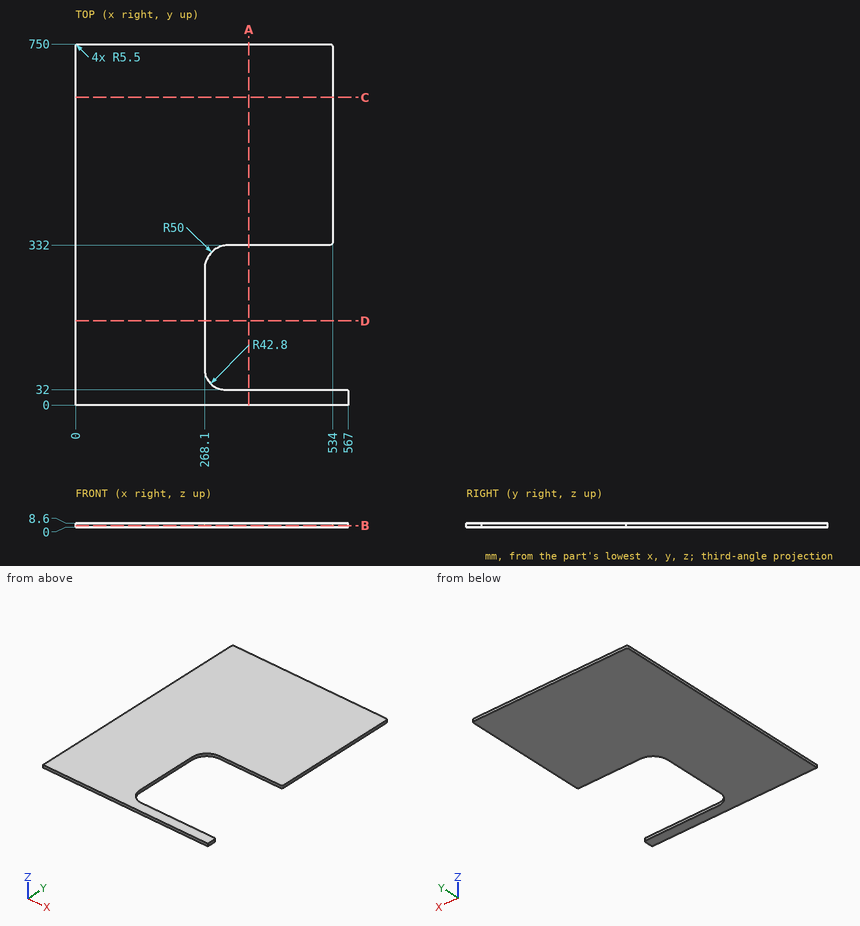
Print and shaded views of the part. All mm, measured from the part's lowest x, y and z. Coordinates: 2 decimals unless noted, no trailing zeros. Order: outer loops, then holes, each group sorted by start corner. A loop starts at its lowest first (then second) coordinate and runs counter-clockwise, first axis right, second up.
Item 1: Drill centre lines: L1, parallel to Y at x = 348, z = 6.75; L2, parallel to X at y = 92, z = 6.5; L3, parallel to X at y = 350, z = 7.5. Where is each one in solid material? Low to high.
Filled in:
L1: y = 0 to 32, 332 to 750
L2: x = 0 to 268.1
L3: x = 0 to 534
Item 2: Saw through at A-A on x = 360. List the corners of the cut face in (y, z), then the cut area to 3 significant figures.
Filled in:
outline: (0, 0) - (32, 0) - (32, 8.6) - (0, 8.6) - close; (332, 0) - (750, 0) - (750, 8.6) - (332, 8.6) - close
area: 3,870 mm2
Item 3: Saw through at C-C on y = 639. List the corners of the cut face in (x, z).
Filled in:
outline: (0, 0) - (534, 0) - (534, 8.6) - (0, 8.6) - close
Item 4: Drop flat-ended pins along their axis: pin 1 Ø4.5 at (y, z) = (502, 3.5) entering from +X; pin 2 Ø2 at (x, z) = (105.5, 7) entering from -Y; pin 3 Ø4.5 at (y, z) = (165.5, 3) entering from +X. Give the stop position or say it passes through.
Filled in:
pin 1: stops at x = 534
pin 2: stops at y = 0
pin 3: stops at x = 268.1
Item 5: Saw through at D-D on y = 175. List the corners of the cut face in (x, z).
Filled in:
outline: (0, 0) - (268.1, 0) - (268.1, 8.6) - (0, 8.6) - close
Item 6: Saw through at B-B on z = 3. List the corners of the cut face in (x, y), then the cut area to 3 significant figures.
Filled in:
outline: (0, 0) - (567, 0) - (567, 26.5) arc R5.5 ccw to (561.5, 32) - (310.9, 32) arc R42.8 cw to (268.1, 74.8) - (268.1, 282) arc R50 cw to (318.1, 332) - (528.5, 332) arc R5.5 ccw to (534, 337.5) - (534, 744.5) arc R5.5 ccw to (528.5, 750) - (5.5, 750) arc R5.5 ccw to (0, 744.5) - close
area: 323,000 mm2
